Input: part model. Units: mm. Frame: model coordinates. A direction names the side the tool comes from. Coordinates: 2 decimals unless noted, no trailing zeros. Order: outer loops, then holes, each group sorted by start corner. A loop starts at its lowest first (then second) coordinate and runs counter-clockwise, first axis right, second up.
Autodesk Inventor part; units mm, degrees
ref_plane "YZ Plane" through (0, 0, 0) normal (1, 0, 0) x (0, 1, 0)
ref_plane "XZ Plane" through (0, 0, 0) normal (0, 1, 0) x (-1, 0, 0)
ref_plane "XY Plane" through (0, 0, 0) normal (0, 0, 1) x (1, 0, 0)
sketch "Sketch1" plane through (0, 0, 0) normal (0, 0, 1) x (1, 0, 0)
  line L0 (16.2, 0) -> (86.2, 0)
  line L1 (86.2, 0) -> (86.2, -32.4)
  line L2 (86.2, -32.4) -> (16.2, -32.4)
  circle A0 centre (16.2, -16.2) radius 5
  circle A1 centre (59.2, -16.2) radius 2
  circle A2 centre (74.2, -16.2) radius 2
  arc A3 (16.2, 0) -> (16.2, -32.4) centre (16.2, -16.2) ccw
  point P0 (0, 0)
  dimension "d1" = 32.4
  dimension "d2" = 10
  dimension "d4" = 16.2
  dimension "d5" = 4
  dimension "d6" = 43
  dimension "d7" = 4
  dimension "d8" = 15
  dimension "d9" = 32.4
extrude "Extrusion1" add sketch "Sketch1" along normal blind 32.4
sketch "Sketch2" plane through (86.2, -32.4, 0) normal (1, 0, 0) x (0, 0, -1)
  line L0 (0, 32.4) -> (-32.4, 32.4)
  line L1 (0, 0) -> (0, 32.4)
  line L2 (-26.45, 5.95) -> (-5.95, 5.95)
  line L3 (-5.95, 5.95) -> (-5.95, 26.45)
  line L4 (-5.95, 26.45) -> (-26.45, 26.45)
  line L5 (-26.45, 26.45) -> (-26.45, 5.95)
  line L6 (-26.45, 5.95) -> (-5.95, 26.45) construction
  line L7 (-5.95, 5.95) -> (-26.45, 26.45) construction
  dimension "d12" = 20.5
  dimension "d13" = 20.5
extrude "Extrusion2" cut sketch "Sketch2" against normal blind 50
sketch "Sketch3" plane through (0, 0, 32.4) normal (0, 0, 1) x (1, 0, 0)
  circle A0 centre (16.2, -16.2) radius 5
  circle A1 centre (16.2, -16.2) radius 11.03
  point P0 (0, 0)
  dimension "d16" = 22.06
extrude "Extrusion3" cut sketch "Sketch3" against normal blind 7.2
fillet "Fillet1" radius 2 10 edges at (0, -16.2, 32.4) (51.2, -32.4, 32.4) (51.2, 0, 32.4) (0, -16.2, 0) (51.2, -32.4, 0) (51.2, 0, 0) (86.2, 0, 16.2) (86.2, -16.2, 32.4) (86.2, -16.2, 0) (86.2, -32.4, 16.2)
properties part number "băng chuyền"
Item 1: Access query for faces 4 (the face through (62, -16, 26.45)), 5 (the face through (26.72, -12.89, 28.85)), 6 (the face through (0.004, -16.556, 16.001)). Directions: +Z, -Z, +X, -X, +Y, -Y. A direction counts if a zero-diameter tool reaches every point of the face in a straight line with its end or side. Return the directions, or none.
Response values:
face 4: +X
face 5: +Z
face 6: +Z, -Z, -X
Item 2: Cut plane C-C on y = -16.2. Count the separate pieces of the cut face and the enclosed holes in it, then the cut area to 3 significant figures.
Response values:
separate pieces: 6
enclosed holes: 0
area: 1,260 mm2
Item 3: Cut plane D-D on x = 74.5. Return loops of the section in (y, z), then the cut area to 3 significant figures.
Response values:
outline: (-32.4, 2) arc R2 ccw to (-30.4, 0) - (-18.18, 0) - (-18.18, 5.95) - (-26.45, 5.95) - (-26.45, 26.45) - (-18.18, 26.45) - (-18.18, 32.4) - (-30.4, 32.4) arc R2 ccw to (-32.4, 30.4) - close; (-14.22, 0) - (-2, 0) arc R2 ccw to (0, 2) - (0, 30.4) arc R2 ccw to (-2, 32.4) - (-14.22, 32.4) - (-14.22, 26.45) - (-5.95, 26.45) - (-5.95, 5.95) - (-14.22, 5.95) - close
area: 579 mm2
Item 4: Ray query, probe 1 along Y at (x, z) = (61.5, 24); probe 2 along X at (y, z) = (-16, 28); probe 3 along Z at (x, y) = (75, -6.5). Return the intervals inside material, ascending.
Response values:
probe 1: y = -32.4 to -26.45, -5.95 to 0
probe 2: x = 0 to 5.17, 27.23 to 57.21, 61.19 to 72.21, 76.19 to 86.2
probe 3: z = 0 to 5.95, 26.45 to 32.4
Item 5: Draft query along Y for faces 1 (the face through (49.72, -0.6, 31.83)), 2 (the face through (51, -32.4, 16)), 3 (the face through (72.202, -16.288, 2.933)). Return one class per face: pulls with the +Y half, pulls with the -Y half, needs draft (parallel to the pull), parting line crosses it, or undercut.
Response values:
face 1: pulls with the +Y half
face 2: pulls with the -Y half
face 3: undercut
Item 6: Pin query (flat end, axial travel): pin 1 Ø6 at (y, z) = (-13.5, 12.5) entering from +X; pin 2 Ø2.5 at (x, y) = (74.2, -16.2) entering from +Z; pin 3 Ø6.5 at (x, y) = (11, -12.5) entering from +Z; pin 4 Ø2 at (y, z) = (-9, 6) entering from -X. Return the tip coordinate at first contact, or that it passes through.
Response values:
pin 1: stops at x = 36.2
pin 2: passes through
pin 3: stops at z = 25.2
pin 4: stops at x = 1.23
Item 7: Cut plane B-B on x = 59.2. Return loops of the section in (y, z).
Response values:
outline: (-32.4, 2) arc R2 ccw to (-30.4, 0) - (-18.2, 0) - (-18.2, 5.95) - (-26.45, 5.95) - (-26.45, 26.45) - (-18.2, 26.45) - (-18.2, 32.4) - (-30.4, 32.4) arc R2 ccw to (-32.4, 30.4) - close; (-14.2, 0) - (-2, 0) arc R2 ccw to (0, 2) - (0, 30.4) arc R2 ccw to (-2, 32.4) - (-14.2, 32.4) - (-14.2, 26.45) - (-5.95, 26.45) - (-5.95, 5.95) - (-14.2, 5.95) - close
Item 8: Cut plane A-A on z = 18. Return loops of the section in (x, y).
Response values:
outline: (16.2, -32.4) - (84.2, -32.4) arc R2 ccw to (86.2, -30.4) - (86.2, -26.45) - (36.2, -26.45) - (36.2, -5.95) - (86.2, -5.95) - (86.2, -2) arc R2 ccw to (84.2, 0) - (16.2, 0) arc R16.2 ccw to start; hole circle Ø10 at (16.2, -16.2)
